```python
from build123d import *

# Parameters (mm, degrees)
SKETCH1_W           = 35
SKETCH1_H           = 8
BOSS_EXTRUDE1_DEPTH = 11
CUT_EXTRUDE1_REACH  = 10
SKETCH2_W           = 15
SKETCH2_H           = 6.5
CUT_EXTRUDE2_REACH  = 10
SKETCH5_W           = 7
SKETCH5_H           = 8
CUT_EXTRUDE4_REACH  = 5
SKETCH7_R           = 1.5
FILLET1_R           = 0.5


with BuildPart() as part:
    # Sketch1 → Boss-Extrude1 (new body)
    with BuildSketch(Plane.XY):
        with Locations((-12, -20.425)):
            Rectangle(SKETCH1_W, SKETCH1_H)
    extrude(amount=BOSS_EXTRUDE1_DEPTH)

    # Sketch2 → Cut-Extrude1 (cut, up to next)
    with BuildSketch(Plane(origin=(0, -24.425, 0), x_dir=(-1, 0, 0), z_dir=(0, -1, 0)), mode=Mode.PRIVATE) as cut_extrude1_sk1:
        with Locations((12, -3.25)):
            Rectangle(SKETCH2_W, SKETCH2_H)
    cut_extrude1_tool1 = extrude(cut_extrude1_sk1.sketch, amount=-CUT_EXTRUDE1_REACH, mode=Mode.PRIVATE) & part.part
    add(cut_extrude1_tool1.solids().sort_by_distance((-12, -24.425, 3.25))[0], mode=Mode.SUBTRACT)

    # Sketch5 → Cut-Extrude2 (cut, up to next)
    with BuildSketch(Plane(origin=(0, -24.425, 0), x_dir=(-1, 0, 0), z_dir=(0, -1, 0)), mode=Mode.PRIVATE) as cut_extrude2_sk1:
        with Locations((-2, -7)):
            Rectangle(SKETCH5_W, SKETCH5_H)
    cut_extrude2_tool1 = extrude(cut_extrude2_sk1.sketch, amount=-CUT_EXTRUDE2_REACH, mode=Mode.PRIVATE) & part.part
    add(cut_extrude2_tool1.solids().sort_by_distance((2, -24.425, 7))[0], mode=Mode.SUBTRACT)
    # Sketch5 → Cut-Extrude2 (cut, up to next)
    with BuildSketch(Plane(origin=(0, -24.425, 0), x_dir=(-1, 0, 0), z_dir=(0, -1, 0)), mode=Mode.PRIVATE) as cut_extrude2_sk2:
        with Locations((26, -7)):
            Rectangle(SKETCH5_W, SKETCH5_H)
    cut_extrude2_tool2 = extrude(cut_extrude2_sk2.sketch, amount=-CUT_EXTRUDE2_REACH, mode=Mode.PRIVATE) & part.part
    add(cut_extrude2_tool2.solids().sort_by_distance((-26, -24.425, 7))[0], mode=Mode.SUBTRACT)

    # Sketch7 → Cut-Extrude4 (cut, up to next)
    with BuildSketch(Plane.XY.offset(3), mode=Mode.PRIVATE) as cut_extrude4_sk1:
        with Locations((2, -20.425)):
            Circle(SKETCH7_R)
    cut_extrude4_tool1 = extrude(cut_extrude4_sk1.sketch, amount=-CUT_EXTRUDE4_REACH, mode=Mode.PRIVATE) & part.part
    add(cut_extrude4_tool1.solids().sort_by_distance((2, -20.425, 3))[0], mode=Mode.SUBTRACT)
    # Sketch7 → Cut-Extrude4 (cut, up to next)
    with BuildSketch(Plane.XY.offset(3), mode=Mode.PRIVATE) as cut_extrude4_sk2:
        with Locations((-26, -20.425)):
            Circle(SKETCH7_R)
    cut_extrude4_tool2 = extrude(cut_extrude4_sk2.sketch, amount=-CUT_EXTRUDE4_REACH, mode=Mode.PRIVATE) & part.part
    add(cut_extrude4_tool2.solids().sort_by_distance((-26, -20.425, 3))[0], mode=Mode.SUBTRACT)

    # Fillet1
    fillet1_edges = [part.edges().sort_by_distance(p)[0] for p in [
        (-24.5, -16.425, 0),
        (0.5, -24.425, 0),
        (-19.5, -20.425, 0),
        (-19.5, -20.425, 6.5),
        (-4.5, -20.425, 6.5),
        (-4.5, -20.425, 0),
        (-19.5, -24.425, 3.25),
        (-4.5, -24.425, 3.25),
        (-12, -24.425, 6.5),
        (-19.5, -16.425, 3.25),
        (-12, -16.425, 6.5),
        (-4.5, -16.425, 3.25),
        (-12, -24.425, 11),
        (-12, -16.425, 11),
        (-29.5, -16.425, 1.5),
        (5.5, -24.425, 1.5),
        (-29.5, -24.425, 1.5),
        (5.5, -20.425, 3),
        (-1.5, -20.425, 3),
        (-1.5, -20.425, 11),
        (-1.5, -24.425, 7),
        (2, -24.425, 3),
        (2, -16.425, 3),
        (-1.5, -16.425, 7),
        (-29.5, -20.425, 3),
        (-22.5, -20.425, 11),
        (-26, -24.425, 3),
        (-22.5, -24.425, 7),
        (-22.5, -16.425, 7),
        (-26, -16.425, 3),
        (0.5, -16.425, 0),
        (5.5, -20.425, 0),
        (-24.5, -24.425, 0),
        (-29.5, -20.425, 0),
    ]]
    fillet(fillet1_edges, radius=FILLET1_R)


solid = part.part
```
Design review of the part built by this model. Coordinates are the model's own, in mm. A direction names the side the tool comes from. Coordinates: 2 decimals unless noted, no trailing zeros. Loops run counter-clockwise (first coordinate to the right, second up) from the corner with the lowest first, then second, coordinate; pieces in that order, holes last. Notation, with made-up numbers: M 19,-8 L 50,-8 A14 ccw 50,0 Z; hole C -16,3.5 d3. An arc over 180 degrees is marked long. One line per question, with ' | ' between items.
(1) Draft analysis for pull direction Y (two halves, no side actions). For faces 1 (the face through (-27.106, -19.411, 1.521)), 2 (the face through (0.894, -19.411, 1.521)), 3 (the face through (-22.5, -20, 7)), 4 (the face through (-11.8, -16.425, 7.3)), state which applies: released by +Y, released by -Y, zero draft, split by the parting line, or undercut.
Filled in:
face 1: undercut | face 2: undercut | face 3: zero draft | face 4: released by +Y
(2) Machinability: for faces 5 (the face through (-1.5, -20, 7)), 6 (the face through (-4.5, -20, 3)), 7 (the face through (-24.56, -19.6, 0)), 8 (the face through (-24, -20, 3)), which of the approach directions +Z, -Z, +X, -X, +Y, -Y give a long, thin tool a straight path to every point of the face, cutting with its end or side? Answer none if there is none.
Filled in:
face 5: +Z, +X, +Y, -Y | face 6: -Z, +Y, -Y | face 7: -Z, +X, -X, +Y, -Y | face 8: +Z, -X, +Y, -Y
(3) We need section C-C (y = -23). Give the boundary of the cut face in (x, z).
Filled in:
outline: M -29.5,0.5 A0.5 ccw -29,0 L -20,0 A0.5 ccw -19.5,0.5 L -19.5,6 A0.5 cw -19,6.5 L -5,6.5 A0.5 cw -4.5,6 L -4.5,0.5 A0.5 ccw -4,0 L 5,0 A0.5 ccw 5.5,0.5 L 5.5,2.5 A0.5 ccw 5,3 L -1,3 A0.5 cw -1.5,3.5 L -1.5,10.5 A0.5 ccw -2,11 L -22,11 A0.5 ccw -22.5,10.5 L -22.5,3 L -29,3 A0.5 ccw -29.5,2.5 Z
(4) We need section D-D (x = -24). Give the boundary of the cut face in (y, z) (3 decimals).
Filled in:
outline: M -24.425,0.5 A0.5 ccw -23.925,0 L -16.925,0 A0.5 ccw -16.425,0.5 L -16.425,2.5 A0.5 ccw -16.925,3 L -23.925,3 A0.5 ccw -24.425,2.5 Z
(5) For pin 1 Ø1.6 at (y, z) = (-22, 4.5) entering from -X, flat-tipped, find the tip position at first contact; note if it passes through.
Filled in:
pin 1: stops at x = -22.5
(6) Wall thickness on probe 1 along Y at (x, z) = (2, 1.75) (3 decimals); probe 2 along X at (y, z) = (-22.75, 1.75); probe 3 along X at (y, z) = (-23, 6): over which ranges is each line inside the solid? List them lowest first.
Filled in:
probe 1: y = -24.425 to -21.925, -18.925 to -16.425 | probe 2: x = -29.5 to -19.5, -4.5 to 5.5 | probe 3: x = -22.5 to -19.5, -4.5 to -1.5
(7) We need section A-A (x = 2). Give the boundary of the cut face in (y, z) (3 decimals).
Filled in:
outline: M -24.425,0.5 A0.5 ccw -23.925,0 L -21.925,0 L -21.925,3 L -23.925,3 A0.5 ccw -24.425,2.5 Z; M -18.925,0 L -16.925,0 A0.5 ccw -16.425,0.5 L -16.425,2.5 A0.5 ccw -16.925,3 L -18.925,3 Z
(8) We need section B-B (z = 4). Give the boundary of the cut face in (x, y) (3 decimals).
Filled in:
outline: M -22.5,-23.925 A0.5 ccw -22,-24.425 L -20,-24.425 A0.5 ccw -19.5,-23.925 L -19.5,-16.925 A0.5 ccw -20,-16.425 L -22,-16.425 A0.5 ccw -22.5,-16.925 Z; M -4.5,-23.925 A0.5 ccw -4,-24.425 L -2,-24.425 A0.5 ccw -1.5,-23.925 L -1.5,-16.925 A0.5 ccw -2,-16.425 L -4,-16.425 A0.5 ccw -4.5,-16.925 Z
